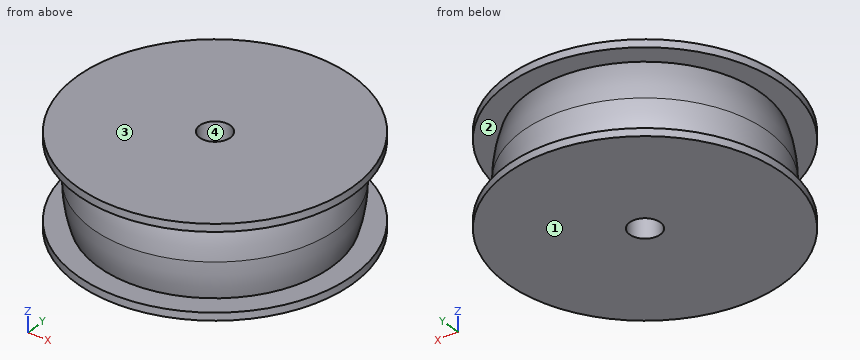
from build123d import *

# Parameters (mm, degrees)
SKETCH5_R          = 1
CUT_EXTRUDE1_DEPTH = 15.071247279


with BuildPart() as part:
    # Sketch1 → Revolve1 (revolve)
    with BuildSketch(Plane(origin=(0, 0, 0), x_dir=(0, 0, -1), z_dir=(1, 0, 0)), mode=Mode.PRIVATE) as revolve1_sk:
        with BuildLine():
            Line((0, 0), (0, 8))
            ThreePointArc((0, 8), (-1.265950905, 7.899200485), (-2.5, 7.599342077))
            Line((-2.5, 7.599342077), (-2.5, 8))
            Line((-2.5, 8), (-2.5, 9))
            Line((-2.5, 9), (-3, 9))
            Line((-3, 9), (-3, 0))
            Line((-3, 0), (0, 0))
        make_face()
        with BuildLine():
            ThreePointArc((2.5, 7.599342077), (1.265950905, 7.899200485), (0, 8))
            Line((0, 8), (0, 0))
            Line((0, 0), (3, 0))
            Line((3, 0), (3, 9))
            Line((3, 9), (2.5, 9))
            Line((2.5, 9), (2.5, 8))
            Line((2.5, 8), (2.5, 7.599342077))
        make_face()
    revolve(revolve1_sk.sketch.rotate(Axis((0, 0, 8.025320303), (0, 0, -1)), 90), axis=Axis((0, 0, 8.025320303), (0, 0, -1)))

    # Sketch5 → Cut-Extrude1 (cut, through all)
    with BuildSketch(Plane.XY.offset(3)):
        Circle(SKETCH5_R)
    extrude(amount=-CUT_EXTRUDE1_DEPTH, mode=Mode.SUBTRACT)


solid = part.part
Geometry check sheet. Reference: the model listing, model coordinates, mm. Face numbers are marked on the shaded views. A direction names the side the tool comes from. Give positions to 0.01 mm unless a question says otherwise; leave off trailing zeros. Write each loop counter-clockwise with the first axis right and the second up, starting at its lowest first coordinate (ties: lowest second). Pieces come first, ordered by that corner, then holes. Notation, with made-up numbers: (45, 30.5) - (98, 30.5) arc R18 cw to (98, 38.5) - close; hole circle Ø10 at (79, 17). An arc over 180 degrees is marked (long way). Put each result on its own line as item: value.
1. Go/stop test with flat-tipped pins: pin 1 (2 mm diameter, centred on x = -6.5, z = 1, fed in from +Y); pin 2 (2.5 mm diameter, centred on x = 0, y = 0, fed in from +Z). Record where each tip stops, or that it passes through.
Ans:
pin 1: stops at y = 5.74
pin 2: stops at z = 3
2. Sectioned sample at C-C, the plane x = -1.5. Enter the section's corners in (y, z), plus the area to 3 significant figures.
Ans:
outline: (-8.87, -3) - (8.87, -3) - (8.87, -2.5) - (7.45, -2.5) arc R7.86 ccw to (7.45, 2.5) - (8.87, 2.5) - (8.87, 3) - (-8.87, 3) - (-8.87, 2.5) - (-7.45, 2.5) arc R7.86 ccw to (-7.45, -2.5) - (-8.87, -2.5) - close
area: 95.0 mm²
3. Sectioned sample at D-D, the plane z = 0.45. Enter the section's corners in (x, y), plus the area to 3 significant figures.
Ans:
outline: circle Ø15.97 at (0, 0); hole circle Ø2 at (0, 0)
area: 197 mm²
4. Thickness scan on line 1 (Z direction, x = 8, y = 2); line 2 (Y direction, x = 0, z = 0.1); line 3 (Y direction, x = 0, z = 1.15). Record the ranges inside material, lowest first.
Ans:
line 1: z = -3 to -2.5, 2.5 to 3
line 2: y = -8 to -1, 1 to 8
line 3: y = -7.92 to -1, 1 to 7.92
5. Sectioned sample at A-A, the plane y = 0. Enter the section's corners in (x, z), plus the area to 3 significant figures.
Ans:
outline: (-9, -3) - (-1, -3) - (-1, 3) - (-9, 3) - (-9, 2.5) - (-7.6, 2.5) arc R8 ccw to (-7.6, -2.5) - (-9, -2.5) - close; (1, -3) - (9, -3) - (9, -2.5) - (7.6, -2.5) arc R8 ccw to (7.6, 2.5) - (9, 2.5) - (9, 3) - (1, 3) - close
area: 84.7 mm²
6. Draft check along Y on the marked faces 3 and 4. Enter one of: +Y half, -Y half, draft (parallel to the pull), parting line (faces both ways), or undercut.
Ans:
face 3: draft
face 4: undercut
7. Set-up check for the marked faces 1 and 2: record each of +Z, -Z, +X, -X, +Y, -Y from which the full face is reachable in a straight line by a thin tool's end or side.
Ans:
face 1: -Z, +X, -X, +Y, -Y
face 2: none
8. Sectioned sample at B-B, the plane x = 8.25. Enter the section's corners in (y, z), plus the area to 3 significant figures.
Ans:
outline: (-3.6, -3) - (3.6, -3) - (3.6, -2.5) - (-3.6, -2.5) - close; (-3.6, 2.5) - (3.6, 2.5) - (3.6, 3) - (-3.6, 3) - close
area: 7.19 mm²
